from build123d import *

# Parameters (mm, degrees)
SKETCH1_W               = 50.8
SKETCH1_H               = 292.1
EXTRUDE1_DEPTH          = 12.7
F_3_8_CLEARANCE_HOLE1_D = 10.31748
SKETCH4_R               = 9.525
CUT_EXTRUDE1_DEPTH      = 297.756364717


with BuildPart() as part:
    # Sketch1 → Extrude1 (new body)
    with BuildSketch(Plane(origin=(0, 0, 0), x_dir=(1, 0, 0), z_dir=(0, 1, 0))):
        with Locations((25.4, 146.05)):
            Rectangle(SKETCH1_W, SKETCH1_H)
    extrude(amount=EXTRUDE1_DEPTH)

    # 3/8 Clearance Hole1 (through all)
    with Locations(Plane(origin=(0, 12.7, 0), x_dir=(-1, 0, 0), z_dir=(0, 1, 0))):
        with Locations((-25.4, -69.85), (-25.4, -222.25)):
            Hole(F_3_8_CLEARANCE_HOLE1_D / 2)

    # Sketch4 → Cut-Extrude1 (cut, through all)
    with BuildSketch(Plane.XZ):
        with Locations(Location((25.4, -146.05, 0), (0, 0, 270))):
            Circle(SKETCH4_R)
    extrude(amount=-CUT_EXTRUDE1_DEPTH, mode=Mode.SUBTRACT)


solid = part.part
Part model, mm, in its own coordinate system. Round coordinates to 2 decimals unless told otherwise and drop trailing zeros. Loops run counter-clockwise (first coordinate to the right, second up) from the corner with the lowest first, then second, coordinate; pieces in that order, holes last. Notation, with made-up numbers: (18.5, 66) - (71.5, 66) arc R20 ccw to (71.5, 73) - close; hole circle Ø5 at (52, 42). An arc over 180 degrees is marked (long way). Answer as a JSON object with one key per item and string values.
Item 1: Band-saw the part on B-B on x = 25.4. List the corners of the cut face in (y, z) (3 decimals), plus the area to 3 significant figures.
Output:
{"outline": "(0, -292.1) - (12.7, -292.1) - (12.7, -227.409) - (0, -227.409) - close; (0, -217.091) - (12.7, -217.091) - (12.7, -155.575) - (0, -155.575) - close; (0, -136.525) - (12.7, -136.525) - (12.7, -75.009) - (0, -75.009) - close; (0, -64.691) - (12.7, -64.691) - (12.7, 0) - (0, 0) - close", "area": "3,210 mm2"}
Item 2: Band-saw the part on A-A on z = -146.05. List the corners of the cut face in (x, y) (3 decimals).
Output:
{"outline": "(0, 0) - (15.875, 0) - (15.875, 12.7) - (0, 12.7) - close; (34.925, 0) - (50.8, 0) - (50.8, 12.7) - (34.925, 12.7) - close"}
Item 3: Band-saw the part on C-C on y = 3. List the corners of the cut face in (x, z) (3 decimals).
Output:
{"outline": "(0, -292.1) - (50.8, -292.1) - (50.8, 0) - (0, 0) - close; hole circle Ø19.05 at (25.4, -146.05); hole circle Ø10.317 at (25.4, -222.25); hole circle Ø10.317 at (25.4, -69.85)"}
Item 4: Band-saw the part on D-D on z = -69.85. List the corners of the cut face in (x, y), plus the area to 3 significant figures.
Output:
{"outline": "(0, 0) - (20.24, 0) - (20.24, 12.7) - (0, 12.7) - close; (30.56, 0) - (50.8, 0) - (50.8, 12.7) - (30.56, 12.7) - close", "area": "514 mm2"}
Item 5: Pin check, flat tip, straight feed: pin 1 (1.5 mm diameter, centred on x = 34.5, y = 1.5, fed in from +Z). Stop position of the tip, or through.
Output:
{"pin 1": "z = 0"}
Item 6: Wall check: L1, parallel to X at y = 7, z = -146.05 (3 decimals); L2, parallel to X at y = 9, z = -70; L3, parallel to Z at x = 32.5, y = 5. Give the ranges that are in metal, low to high.
Output:
{"L1": "0 to 15.875, 34.925 to 50.8", "L2": "0 to 20.24, 30.56 to 50.8", "L3": "-292.1 to -152.4, -139.7 to 0"}
Item 7: Pull direction X, two halves, no side cores. Call faces 1 (the face through (0, 6, -144)), 2 (the face through (50.8, 6, -144)), 3 (the face through (36, 12.7, -148)), 4 (the face through (27.78, 6.261, -226.827)): pulls with the +X half, pulls with the -X half, needs draft (parallel to the pull), parting line crosses it, or undercut.
Output:
{"face 1": "pulls with the -X half", "face 2": "pulls with the +X half", "face 3": "needs draft", "face 4": "undercut"}
